CAD build for the part. Positions are in the model's coordinates, mm. A direction names the side the tool comes from. Give positions to 0.01 mm unless a question says otherwise; leave off trailing zeros. Order: outer loops, then holes, each group sorted by start corner. A loop starts at its lowest first (then second) coordinate and runs counter-clockwise, first axis right, second up. Notation, with made-up numbers: M 42,11.25 L 48,11.25 A19 cw 48,24.25 Z; hole C 46,-4.75 d8. An arc over 180 degrees is marked long. Put each result on its own line as item: value. Start each with the question number.
1) Cut at C-C (x = -16). Write the cut outline in (y, z), and give its area (3 significant figures).
2) Cut at A-A (x = 2.05). Write the cut outline in (y, z).
3) Tool access for faces 4 (the face through (43, 1, -10)), 5 (the face through (-10, 3.6, -7)), 6 (the face through (44, 6, -4.25)), 7 (the face through (-9.9, 3.2, -9.7)): list every direction of +Z, -Z, +X, -X, +Y, -Y with a clear straight run to the whole face (end or side of a thin tool).
4) Two-plate mould, pull along X, no slides. Class faces 1 (the face through (41.88, 0.79, -1.61)), 2 (the face through (21, 0, -11)), 3 (the face through (0, 1, -1)): released by +X, released by -X, zero draft, split by the parting line, or undercut.
5) Cut at D-D (y = 9.25). Write the cut outline in (x, z).
6) Cut at B-B (z = -18.8). Write the cut outline in (x, y), and give its area (3 significant figures).
7) Drill centre lines: line 1 (X direction, y = 0.7, z = -18.8); line 2 (X direction, y = 3, z = -12); line 3 (Z direction, x = 46, y = 2.25). Where is each one in solid material? Low to high. Write a range as [from, to].
8) Pin check, flat tips, straight feed: pin 1 (5 mm diameter, centred on x = 23.5, z = -3, fed in from +Y); pin 2 (3 mm diameter, centred on x = -12.5, z = -15, fed in from +Y); pin 3 (4 mm diameter, centred on x = -7.5, y = 1.5, fed in from +Z). Stop position of each tip, or through.
```python
from build123d import *

# Parameters (mm, degrees)
SKETCH1_W           = 43
SKETCH1_H           = 21
SKETCH1_R           = 1.1
BOSS_EXTRUDE1_DEPTH = 1.6
BOSS_EXTRUDE2_DEPTH = 20
SKETCH3_W           = 13.2
SKETCH3_H           = 12.5
BOSS_EXTRUDE3_DEPTH = 9


with BuildPart() as part:
    # Sketch1 → Boss-Extrude1 (new body)
    with BuildSketch(Plane(origin=(0, 0, 0), x_dir=(1, 0, 0), z_dir=(0, 1, 0))):
        with Locations((21.5, 10.5)):
            Rectangle(SKETCH1_W, SKETCH1_H)
        with Locations(Location((2.05, 18.8, 0), (0, 0, 270))):
            Circle(SKETCH1_R, mode=Mode.SUBTRACT)
        with Locations(Location((40.95, 18.8, 0), (0, 0, 270))):
            Circle(SKETCH1_R, mode=Mode.SUBTRACT)
        with Locations(Location((40.95, 2.2, 0), (0, 0, 270))):
            Circle(SKETCH1_R, mode=Mode.SUBTRACT)
        with Locations(Location((2.05, 2.2, 0), (0, 0, 270))):
            Circle(SKETCH1_R, mode=Mode.SUBTRACT)
    extrude(amount=BOSS_EXTRUDE1_DEPTH)

    # Sketch2 → Boss-Extrude2 (add)
    with BuildSketch(Plane.ZY):
        with BuildLine():
            ThreePointArc((-16, 3.6), (-17.414213562, 3.014213562), (-18, 1.6))
            Line((-18, 1.6), (-11, 1.6))
            ThreePointArc((-11, 1.6), (-10.875, 1.930718914), (-10.5625, 2.096078371))
            ThreePointArc((-10.5625, 2.096078371), (-11.273655175, 3.179898215), (-12.5, 3.6))
            Line((-12.5, 3.6), (-16, 3.6))
        make_face()
        with BuildLine():
            Line((-17.2, 0), (-11.3, 0))
            ThreePointArc((-11.3, 0), (-10.836979464, 0.488981235), (-10.5625, 1.103921629))
            ThreePointArc((-10.5625, 1.103921629), (-10.875, 1.269281086), (-11, 1.6))
            Line((-11, 1.6), (-18, 1.6))
            ThreePointArc((-18, 1.6), (-17.788854382, 0.705572809), (-17.2, 0))
        make_face()
        with BuildLine():
            Line((-16, -0.4), (-12.5, -0.4))
            ThreePointArc((-12.5, -0.4), (-11.867544468, -0.297366596), (-11.3, 0))
            Line((-11.3, 0), (-17.2, 0))
            ThreePointArc((-17.2, 0), (-16.632455532, -0.297366596), (-16, -0.4))
        make_face()
        with BuildLine():
            ThreePointArc((-11, 1.6), (-10.875, 1.269281086), (-10.5625, 1.103921629))
            ThreePointArc((-10.5625, 1.103921629), (-10.515686517, 1.35), (-10.5, 1.6))
            Line((-10.5, 1.6), (-11, 1.6))
        make_face()
        with BuildLine():
            Line((-11, 1.6), (-10.5, 1.6))
            ThreePointArc((-10.5, 1.6), (-10.515686517, 1.85), (-10.5625, 2.096078371))
            ThreePointArc((-10.5625, 2.096078371), (-10.875, 1.930718914), (-11, 1.6))
        make_face()
        with BuildLine():
            ThreePointArc((-10.5, 1.6), (-10.515686517, 1.35), (-10.5625, 1.103921629))
            ThreePointArc((-10.5625, 1.103921629), (-10.5, 1.1), (-10.4375, 1.103921629))
            ThreePointArc((-10.4375, 1.103921629), (-10.484313483, 1.35), (-10.5, 1.6))
        make_face()
        with BuildLine():
            ThreePointArc((-10.5625, 2.096078371), (-10.515686517, 1.85), (-10.5, 1.6))
            ThreePointArc((-10.5, 1.6), (-10.484313483, 1.85), (-10.4375, 2.096078371))
            ThreePointArc((-10.4375, 2.096078371), (-10.5, 2.1), (-10.5625, 2.096078371))
        make_face()
        with BuildLine():
            Line((-10, 1.6), (-10.5, 1.6))
            ThreePointArc((-10.5, 1.6), (-10.484313483, 1.35), (-10.4375, 1.103921629))
            ThreePointArc((-10.4375, 1.103921629), (-10.125, 1.269281086), (-10, 1.6))
        make_face()
        with BuildLine():
            ThreePointArc((-10.4375, 2.096078371), (-10.484313483, 1.85), (-10.5, 1.6))
            Line((-10.5, 1.6), (-10, 1.6))
            ThreePointArc((-10, 1.6), (-10.125, 1.930718914), (-10.4375, 2.096078371))
        make_face()
        with BuildLine():
            ThreePointArc((-10.4375, 1.103921629), (-10.163020536, 0.488981235), (-9.7, 0))
            Line((-9.7, 0), (-3.8, 0))
            ThreePointArc((-3.8, 0), (-3.211145618, 0.705572809), (-3, 1.6))
            Line((-3, 1.6), (-10, 1.6))
            ThreePointArc((-10, 1.6), (-10.125, 1.269281086), (-10.4375, 1.103921629))
        make_face()
        with BuildLine():
            ThreePointArc((-8.5, 3.6), (-9.726344825, 3.179898215), (-10.4375, 2.096078371))
            ThreePointArc((-10.4375, 2.096078371), (-10.125, 1.930718914), (-10, 1.6))
            Line((-10, 1.6), (-3, 1.6))
            ThreePointArc((-3, 1.6), (-3.585786438, 3.014213562), (-5, 3.6))
            Line((-5, 3.6), (-8.5, 3.6))
        make_face()
        with BuildLine():
            Line((-3.8, 0), (-9.7, 0))
            ThreePointArc((-9.7, 0), (-9.132455532, -0.297366596), (-8.5, -0.4))
            Line((-8.5, -0.4), (-5, -0.4))
            ThreePointArc((-5, -0.4), (-4.367544468, -0.297366596), (-3.8, 0))
        make_face()
    extrude(amount=BOSS_EXTRUDE2_DEPTH)

    # Sketch3 → Boss-Extrude3 (add)
    with BuildSketch(Plane(origin=(0, 1.6, 0), x_dir=(1, 0, 0), z_dir=(0, 1, 0))):
        with Locations((43.9, 10.5)):
            Rectangle(SKETCH3_W, SKETCH3_H)
    extrude(amount=BOSS_EXTRUDE3_DEPTH)


solid = part.part
```
Solution:
1. outline: M -0.4,-16 A2 ccw 3.6,-16 L 3.6,-12.5 A2 ccw 2.1,-10.56 A0.5 ccw 2.1,-10.44 A2 ccw 3.6,-8.5 L 3.6,-5 A2 ccw -0.4,-5 L -0.4,-8.5 A2 ccw 1.1,-10.44 A0.5 ccw 1.1,-10.56 A2 ccw -0.4,-12.5 Z
1. area: 53.2 mm²
2. outline: M 0,-21 L 1.6,-21 L 1.6,-19.9 L 0,-19.9 Z; M 0,-17.7 L 1.6,-17.7 L 1.6,-3.3 L 0,-3.3 Z; M 0,-1.1 L 1.6,-1.1 L 1.6,0 L 0,0 Z
3. face 4: +Z, -Z, +X, -Y
3. face 5: +Z, -Z, -X, +Y
3. face 6: +Z, +X, +Y
3. face 7: -X, +Y
4. face 1: undercut
4. face 2: zero draft
4. face 3: released by -X
5. outline: M 37.3,-16.75 L 50.5,-16.75 L 50.5,-4.25 L 37.3,-4.25 Z
6. outline: M 0,0 L 0.95,0 L 0.95,1.6 L 0,1.6 Z; M 3.15,0 L 39.85,0 L 39.85,1.6 L 3.15,1.6 Z; M 42.05,0 L 43,0 L 43,1.6 L 42.05,1.6 Z
6. area: 61.8 mm²
7. line 1: [0, 0.95], [3.15, 39.85], [42.05, 43]
7. line 2: [-20, 0], [37.3, 50.5]
7. line 3: [-16.75, -4.25]
8. pin 1: y = 1.6
8. pin 2: y = 3.6
8. pin 3: z = -3
